Source: CAD feature listing. Evaluate the final solid. Frame: model axes, mm. A direction names the side the tool comes from. Round coordinates to 2 decimals unless told otherwise and drop trailing zeros. Order: outer loops, then holes, each group sorted by start corner. A loop starts at its lowest first (then second) coordinate and runs counter-clockwise, first axis right, second up. Notation, with made-up numbers: (51.5, 21.25) -> (77.5, 21.25) arc R20 ccw to (77.5, 44.25) -> close; hole circle Ø4 at (-38.75, 75). An arc over 180 degrees is marked (long way). Write item = value, one per line. Start each with the question number.
(1) Reachability of faces 4 (the face through (9.525, 0, 1)), 5 (the face through (-12.7, -1, 1)) from +Z, -Z, +X, -X, +Y, -Y: full face, straight path, thin tool, end or side. Return the list, or none.
(2) Ray query, line 1 (X direction, y = -19, z = -6) (3 decimals); line 2 (Y direction, x = -5.25, z = -2.5) (3 decimals). Return the intervals inside material, ascending.
(3) Draft query along Y for faces 1 (the face through (-10, 3, -61.912)), 2 (the face through (0, -34.925, 1)), 3 (the face through (0, 38.1, 1)). Return one class per face: released by +Y, released by -Y, zero draft, split by the parting line, or undercut.
(4) Cut plane A-A on x = -5.5. Return the cut outline in (y, z) (1 decimal), then the cut area to 3 significant figures.
(5) Cut plane C-C on y = -25. Return the cut outline in (x, z) (1 decimal), then the cut area to 3 significant figures.
(6) Cut plane B-B on z = 9.5. Return the cut outline in (x, y) (3 decimals), then the cut area to 3 significant figures.
from build123d import *

# Parameters (mm, degrees)
SKETCH1_W           = 25.4
SKETCH1_H           = 76.2
BOSS_EXTRUDE1_DEPTH = 61.9125
SHELL1_T            = -3.175


with BuildPart() as part:
    # Sketch1 → Boss-Extrude1 (new body, symmetric)
    with BuildSketch(Plane.XY):
        Rectangle(SKETCH1_W, SKETCH1_H)
    extrude(amount=BOSS_EXTRUDE1_DEPTH, both=True)

    # Shell1
    shell1_openings = [part.faces().sort_by_distance(p)[0] for p in [
        (0, 0, 61.9125),
        (0, 0, -61.9125),
    ]]
    offset(amount=SHELL1_T, openings=shell1_openings, kind=Kind.INTERSECTION)


solid = part.part
Evaluation:
q1.face_4 = +Z, -Z
q1.face_5 = +Z, -Z, -X, +Y, -Y
q2.line_1 = -12.7 to -9.525, 9.525 to 12.7
q2.line_2 = -38.1 to -34.925, 34.925 to 38.1
q3.face_1 = zero draft
q3.face_2 = undercut
q3.face_3 = released by +Y
q4.outline = (-38.1, -61.9) -> (-34.9, -61.9) -> (-34.9, 61.9) -> (-38.1, 61.9) -> close; (34.9, -61.9) -> (38.1, -61.9) -> (38.1, 61.9) -> (34.9, 61.9) -> close
q4.area = 786 mm^2
q5.outline = (-12.7, -61.9) -> (-9.5, -61.9) -> (-9.5, 61.9) -> (-12.7, 61.9) -> close; (9.5, -61.9) -> (12.7, -61.9) -> (12.7, 61.9) -> (9.5, 61.9) -> close
q5.area = 786 mm^2
q6.outline = (-12.7, -38.1) -> (12.7, -38.1) -> (12.7, 38.1) -> (-12.7, 38.1) -> close; hole (-9.525, -34.925) -> (9.525, -34.925) -> (9.525, 34.925) -> (-9.525, 34.925) -> close
q6.area = 605 mm^2
